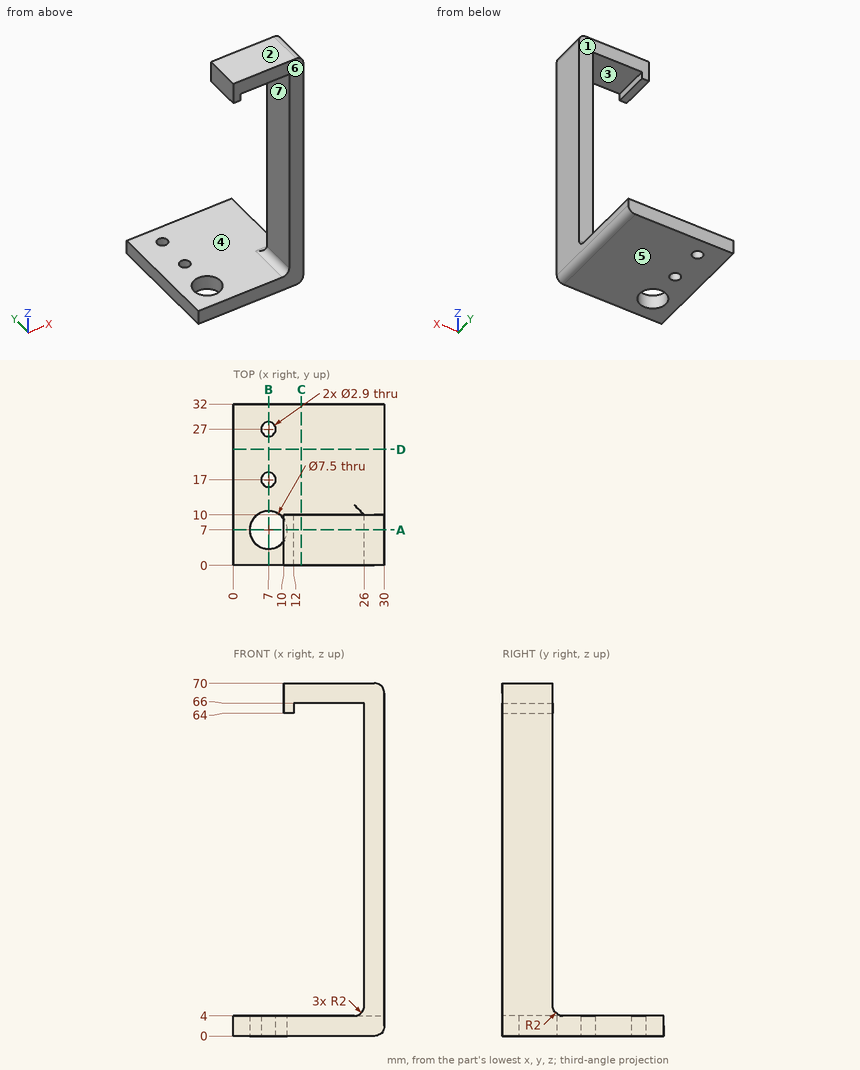
Can you work these out from the drawing? Everything is in mm from the part's minimum corner. A direction names the side the tool comes from. Give positions to 0.01 mm unless a question says otherwise; leave off trailing zeros. Order: outer loops, then holes, each group sorted by start corner. A loop starts at its lowest first (then second) coordinate and runs counter-clockwise, first axis right, second up.
1. Suppose I cut it at C-C (x = 13.5). List the corners of the cut face in (y, z) for me.
2. Suppose I cut it at D-D (y = 23). List the corners of the cut face in (x, z) for me, plus the area to 3 significant figures.
3. I need wall thicknesses on L1, parallel to Y at x = 7, z = 1.4; L2, parallel to Z at x = 13.25, y = 4; L3, parallel to Z at x = 9.75, y = 30. Which ranges of each line are inside material? Lowest first, please.
4. Suppose I cut it at A-A (y = 7). List the corners of the cut face in (x, z) for me.
5. Suppose I cut it at B-B (x = 7). List the corners of the cut face in (y, z) for me, plus the area to 3 significant figures.
6. For the marked faces 1, 2 and 3, which set-ups out of +Z, -Z, +X, -X, +Y, -Y let a thin tool reach every point of the face, with its end or its side?
7. Will these pins go through, and if not, where does the flat tip stop? P1, Ø2, axis at x = 7.5, y = 24.5, coming from the +Z side; P2, Ø3, axis at y = 5, z = 32, coming from the -X side; P3, Ø1.8, axis at y = 5.5, z = 67.5, coming from the -X side.
8. We'd pull the mould along Z, two halves only. Please class the marked faces 4, 5, 6 and 7: pulls with the +Z half, pulls with the -Z half, needs draft (parallel to the pull), parting line crosses it, or undercut.
Solved:
1. outline: (0, 0) - (32, 0) - (32, 4) - (0, 4) - close; (0, 66) - (10, 66) - (10, 70) - (0, 70) - close
2. outline: (0, 0) - (28, 0) arc R2 ccw to (30, 2) - (30, 4) - (0, 4) - close
2. area: 119 mm2
3. L1: y = 0 to 3.25, 10.75 to 15.55, 18.45 to 25.55, 28.45 to 32
3. L2: z = 0 to 4, 66 to 70
3. L3: z = 0 to 4
4. outline: (0, 0) - (3.25, 0) - (3.25, 4) - (0, 4) - close; (10, 64) - (12, 64) - (12, 66) - (26, 66) - (26, 6) arc R2 cw to (24, 4) - (10.75, 4) - (10.75, 0) - (28, 0) arc R2 ccw to (30, 2) - (30, 68) arc R2 ccw to (28, 70) - (10, 70) - close
5. outline: (0, 0) - (3.25, 0) - (3.25, 4) - (0, 4) - close; (10.75, 0) - (15.55, 0) - (15.55, 4) - (10.75, 4) - close; (18.45, 0) - (25.55, 0) - (25.55, 4) - (18.45, 4) - close; (28.45, 0) - (32, 0) - (32, 4) - (28.45, 4) - close
5. area: 74.8 mm2
6. face 1: +Z, +X, -X, +Y
6. face 2: +Z, +X, -X, +Y, -Y
6. face 3: +Y, -Y
7. P1: stops at z = 4
7. P2: stops at x = 26
7. P3: stops at x = 10
8. face 4: undercut
8. face 5: pulls with the -Z half
8. face 6: needs draft
8. face 7: undercut
